Read the model definition and answer for the solid it produces. Units are mm, in the model's axes. A direction names the side the tool comes from. Round coordinates to 2 decimals unless told otherwise and drop trailing zeros. Write each loop counter-clockwise with the first axis right and the second up, starting at its lowest first coordinate (ties: lowest second). Pieces come first, ordered by that corner, then holes. Notation, with made-up numbers: (65.5, 16.25) - (110.5, 16.25) arc R19 cw to (110.5, 49.25) - close; hole circle Ø5 at (-10, 85.5). An arc over 180 degrees is marked (long way). Answer as CSV lines item,"result". Start each with the question number.
1) Consider line 1 along Z through (x, y) = (-478, 2.5); line 2 along Z through (x, y) = (-259.5, -2.5); line 3 along Y through (x, z) = (429, -5). Determine where each line is inside the solid, lowest interval first.
2) Which of the six approach directions +Z, -Z, +X, -X, +Y, -Y give full straight-line access (tool end or side, diameter ignored) to faces 1 (the cylindrical face through (-460.134, 13.267, -12.165)), 2 (the flat face through (540, 0, 0)), 3 (the cylindrical face through (457.866, 13.267, -12.165))?
3) Each of these flat-tipped pins is pushed along its axis until it touches: pin 1 (12 mm diameter, centred on x = 190, y = -25, fed in from -Z); pin 2 (10 mm diameter, centred on x = -286, z = 1, fed in from -Y); pin 3 (1.5 mm diameter, centred on x = 211.5, z = 23, fed in from +Y). Where does it stop, or does it pass through?
4) Find section A-A on x = -474.5. Determine the outline of the cut face in (y, z), then the cut area to 3 significant figures.
5) Find section B-B on x = -39. Determine the outline of the cut face in (y, z), then the cut area to 3 significant figures.
from build123d import *

# Parameters (mm, degrees)
SCALE1_SCALE = 18


with BuildPart() as part:
    # Sketch1 → Revolve1 (revolve)
    with BuildSketch(Plane.XY, mode=Mode.PRIVATE) as revolve1_sk:
        with BuildLine():
            Line((-30, 0), (30, 0))
            Line((30, 0), (30, 1))
            Line((30, 1), (21, 1))
            ThreePointArc((21, 1), (19.881966011, 1.126602828), (18.820550528, 1.5))
            ThreePointArc((18.820550528, 1.5), (17.759135045, 1.873397172), (16.641101056, 2))
            Line((16.641101056, 2), (-16.641101056, 2))
            ThreePointArc((-16.641101056, 2), (-17.759135045, 1.873397172), (-18.820550528, 1.5))
            ThreePointArc((-18.820550528, 1.5), (-19.881966011, 1.126602828), (-21, 1))
            Line((-21, 1), (-30, 1))
            Line((-30, 1), (-30, 0))
        make_face()
    revolve(revolve1_sk.sketch.rotate(Axis((-30, 0, 0), (1, 0, 0)), 180), axis=Axis((-30, 0, 0), (1, 0, 0)))


with BuildPart() as part_1:
    # Scale1: scaled about (0, 0, 0)
    add(part.part.scale(SCALE1_SCALE))


solid = part_1.part
Check values:
1,line 1,"z = -17.83 to 17.83"
1,line 2,"z = -35.91 to 35.91"
1,line 3,"y = -17.29 to 17.29"
2,face 1,"-X"
2,face 2,"+Z, -Z, +X, +Y, -Y"
2,face 3,"+X"
3,pin 1,"stops at z = -30.58"
3,pin 2,"stops at y = -36"
3,pin 3,"stops at y = 28.3"
4,outline,"circle Ø36 at (0, 0)"
4,area,"1,020 mm^2"
5,outline,"circle Ø72 at (0, 0)"
5,area,"4,070 mm^2"
